Here's how the part is built. I have some questions about the finished solid (model axes, mm). Face numbers are marked on the shaded views. A direction names the side the tool comes from. Give positions to 0.01 mm unless a question says otherwise; leave off trailing zeros. Loops run counter-clockwise (first coordinate to the right, second up) from the corner with the lowest first, then second, coordinate; pieces in that order, holes last. Notation, with made-up numbers: (4.25, 2.5) - (11.25, 2.5) arc R15 ccw to (11.25, 16.5) - close; hole circle Ø4 at (-21.75, 53). An arc over 180 degrees is marked (long way). Return JSON: item names as keys, results as strings. Group by question number.
(1) If we mould it in two halves opening along Y, with no side actions, what happens to the marked faces 5, 6 and 7? For each: released by +Y, released by -Y, zero draft, split by the parting line, or undercut.
(2) If we section it at D-D (x = 2): Please give me the cut outline in (y, z), then the cut area to 3 significant figures.
(3) If we section it at C-C (z = 33): Please give me the cut outline in (x, y), then the cut area to 3 significant figures.
(4) If we section it at B-B (y = 26): Please give me the cut outline in (x, z).
(5) On a 3-axis mill with a long thin cutter (end or side, diameter ignored), from which of +Z, -Z, +X, -X, +Y, -Y can I reach the whole of each face in a straight line? I mean the marked faces 1, 2, 3 and 4. Say none if no direction works.
(6) For P1, Ø25, axis at y = 20, z = 34, coming from the -X side; P2, Ø1.5, axis at y = 41.5, z = 30.5, coming from the +X side; P3, Ø9, axis at x = -12.5, y = 29, coming from the -Z side, each with a flat end and sliding along its axis, tell me the tip position at first contact or that it passes through.
(7) If we section it at A-A (x = 21): Please give me the cut outline in (y, z), then the cut area to 3 significant figures.
(8) I need wall thicknesses on probe 1 along Z at (x, y) = (13.75, 26); probe 2 along X at (y, z) = (42, 12.5); probe 3 along X at (y, z) = (34, 21.5). Which ranges of each line are inside material? Lowest first, please. Write a range as [from, to].
Solid Edge part; units mm, degrees
sketch "Sketch1" plane through (0, 0, 0) normal (0, -1, 0) x (1, 0, 0)
  line L0 (-25, 7) -> (-25, 57)
  line L1 (-25, 57) -> (8, 57)
  line L2 (8, 7) -> (8, 57)
  line L3 (30, 7) -> (8, 7)
  line L4 (30, 0) -> (30, 7)
  line L5 (0, 0) -> (30, 0)
  line L6 (0, 50) -> (0, 0)
  line L7 (-18, 50) -> (0, 50)
  line L8 (-18, 0) -> (-18, 50)
  line L9 (-32, 0) -> (-18, 0)
  line L10 (-32, 7) -> (-32, 0)
  line L11 (-32, 7) -> (-25, 7)
extrude "ProtrusiónExtruida_1" add sketch "Sketch1" against normal blind 52
sketch "Sketch2" plane through (19, 26, 7) normal (0, 0, 1) x (0, 1, 0)
  line L0 (-10, -11) -> (10, -11)
  line L1 (10, -11) -> (10, 1)
  line L2 (10, 1) -> (-10, 1)
  line L3 (-10, 1) -> (-10, -11)
extrude "VaciadoExtruido_1" cut sketch "Sketch2" against normal blind 7
sketch "Sketch3" plane through (8, 26, 32) normal (1, 0, 0) x (0, 1, 0)
  circle A0 centre (0, 1) radius 15
extrude "ProtrusiónExtruida_2" add sketch "Sketch3" along normal blind 20
hole "Agujero_1" at (28, 26, 33) direction (-1, 0, 0) diameter 14 end up to next
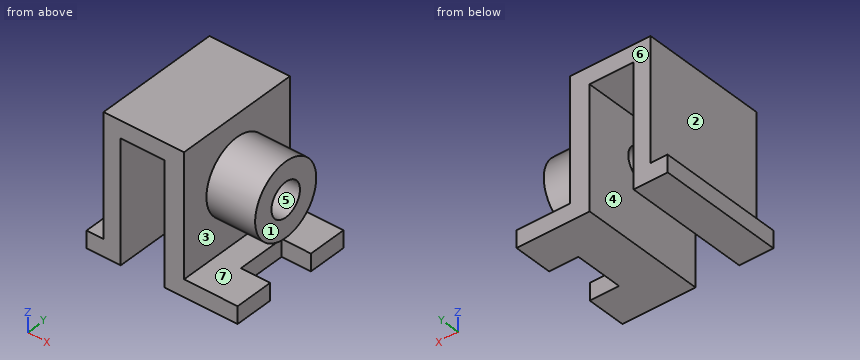
Values:
{
 "1": {"face 5": "undercut", "face 6": "released by +Y", "face 7": "zero draft"},
 "2": {"outline": "(0, 0) - (52, 0) - (52, 57) - (0, 57) - close; hole circle Ø14 at (26, 33)", "area": "2,810 mm2"},
 "3": {"outline": "(-25, 0) - (-18, 0) - (-18, 52) - (-25, 52) - close; (0, 0) - (8, 0) - (8, 11) - (28, 11) - (28, 19) - (0, 19) - close; (0, 33) - (28, 33) - (28, 41) - (8, 41) - (8, 52) - (0, 52) - close", "area": "988 mm2"},
 "4": {"outline": "(-32, 0) - (-18, 0) - (-18, 50) - (0, 50) - (0, 40) - (28, 40) - (28, 48) - (8, 48) - (8, 57) - (-25, 57) - (-25, 7) - (-32, 7) - close; (0, 0) - (18, 0) - (18, 7) - (8, 7) - (8, 18) - (28, 18) - (28, 26) - (0, 26) - close"},
 "5": {"face 1": "+Z, +X, +Y, -Y", "face 2": "+Z, -X, +Y, -Y", "face 3": "+X", "face 4": "-Z, +Y, -Y"},
 "6": {"P1": "x = -25", "P2": "x = 28", "P3": "z = 50"},
 "7": {"outline": "(0, 0) - (16, 0) - (16, 7) - (0, 7) - close; circle Ø30 at (26, 33); (36, 0) - (52, 0) - (52, 7) - (36, 7) - close; hole circle Ø14 at (26, 33)", "area": "777 mm2"},
 "8": {"probe 1": "[0, 7], [18, 26], [40, 48]", "probe 2": "[-25, -18], [0, 8]", "probe 3": "[-25, -18], [0, 28]"}
}
